Build history of the part. All positions in model axes, mm. A direction names the side the tool comes from. Give positions to 0.01 mm unless a question says otherwise; leave off trailing zeros. Order: outer loops, then holes, each group sorted by start corner. A loop starts at its lowest first (then second) coordinate and runs counter-clockwise, first axis right, second up. Notation, with made-up numbers: M 76,15.5 L 126,15.5 A12 ccw 126,33.5 Z; hole C 50,-8.75 d8. An arc over 180 degrees is marked long. Answer as CSV lines item,"result".
from build123d import *

# Parameters (mm, degrees)
F1_R     = 2.05
F2_DEPTH = 60
F3_DEPTH = 45
F4_SIZE  = 1.5


with BuildPart() as f2:
    # F1 (on Front) → F2 (new body, symmetric)
    with BuildSketch(Plane.XZ):
        Polygon((-2.5980762114, -4.5), (2.5980762114, -4.5), (5.1961524227, 0), (2.5980762114, 4.5), (-2.5980762114, 4.5), (-5.1961524227, 0), align=None)
        Circle(F1_R, mode=Mode.SUBTRACT)
    extrude(amount=F2_DEPTH, both=True)

    # F1 (on Front) → F3 (join, symmetric)
    with BuildSketch(Plane.XZ):
        Circle(F1_R)
    extrude(amount=F3_DEPTH, both=True)

    # F4
    f4_edges = [f2.edges().sort_by_distance(p)[0] for p in [
        (3.897114, -60, 2.25),
        (0, -60, 4.5),
        (-3.897114, -60, 2.25),
        (-3.897114, -60, -2.25),
        (0, -60, -4.5),
        (3.897114, -60, -2.25),
        (3.897114, 60, 2.25),
        (0, 60, 4.5),
        (-3.897114, 60, 2.25),
        (-3.897114, 60, -2.25),
        (0, 60, -4.5),
        (3.897114, 60, -2.25),
    ]]
    chamfer(f4_edges, length=F4_SIZE)


solid = f2.part
Item 1: Band-saw the part on B-B (y = 7.5). Give the cut face in (x, z), and give its area (3 significant figures).
Geometry says:
outline,"M -5.2,0 L -2.6,-4.5 L 2.6,-4.5 L 5.2,0 L 2.6,4.5 L -2.6,4.5 Z"
area,"70.1 mm2"
Item 2: Probe line 1 along Z through (x, y) = (0, 48.5); line 2 along Z through (x, y) = (-1.25, -47); line 3 along Y through (x, z) = (1.75, 0.5). List the from-to ranges inside material, lowest first. Write a range as from..to.
Geometry says:
line 1,"z = -4.5..-2.05, 2.05..4.5"
line 2,"z = -4.5..-1.62, 1.62..4.5"
line 3,"y = -45..45"
Item 3: Drop flat-ended pins along their axis: pin 1 (1 mm diameter, centred on x = -4, y = 22.5, fed in from +Z); pin 2 (4 mm diameter, centred on y = 9.5, z = 3, fed in from -X); pin 3 (1 mm diameter, centred on x = -4, z = -1.5, fed in from -Y). Give the stop position or say it passes through.
Geometry says:
pin 1,"stops at z = 2.94"
pin 2,"stops at x = -4.62"
pin 3,"stops at y = -59.29"
Item 4: Band-saw the part on A-A (x = 0). Give the cut face in (y, z), and give its area (4 significant figures).
Geometry says:
outline,"M -60,-3 L -58.5,-4.5 L 58.5,-4.5 L 60,-3 L 60,-2.05 L 45,-2.05 L 45,2.05 L 60,2.05 L 60,3 L 58.5,4.5 L -58.5,4.5 L -60,3 L -60,2.05 L -45,2.05 L -45,-2.05 L -60,-2.05 Z"
area,"952.5 mm2"
Item 5: Pull direction Z, two halves, no side cores. Call faces 4 (the cylindrical face through (-0.267, 52.605, 2.033)), 5 (the flat face through (0, -1, 4.5)), 6 (the flat face through (3.88, -0.82, -2.28)): released by +Z, released by -Z, zero draft, split by the parting line, or undercut.
Geometry says:
face 4,"undercut"
face 5,"released by +Z"
face 6,"released by -Z"
Item 6: 3-axis set-ups, long thin cutter, end or side, ignore diameter. For faces 1 (the flat face through (0, -45, 0)), 2 (the flat face through (3.22, -59.26, -1.9)), 3 (the flat face through (0, 45, 0)): which of +Z, -Z, +X, -X, +Y, -Y reach the whole face in a straight line?
Geometry says:
face 1,"-Y"
face 2,"-Z, +X, -Y"
face 3,"+Y"
